from build123d import *

# Parameters (mm, degrees)
F1_DEPTH = 11.906
F3_DEPTH = 3.81
F5_DEPTH = 14.54711
F7_R     = 0.4


with BuildPart() as f1:
    # F0 (on Front) → F1 (new body)
    with BuildSketch(Plane.XZ):
        with BuildLine():
            Line((5.478281, 8.795274), (-5.478281, 8.795274))
            ThreePointArc((-5.478281, 8.795274), (-6.747731, 8.26945), (-7.273555, 7))
            Line((-7.273555, 7), (-7.273555, -7))
            ThreePointArc((-7.273555, -7), (-6.747731, -8.26945), (-5.478281, -8.795274))
            Line((-5.478281, -8.795274), (5.478281, -8.795274))
            ThreePointArc((5.478281, -8.795274), (6.747731, -8.26945), (7.273555, -7))
            Line((7.273555, -7), (7.273555, 7))
            ThreePointArc((7.273555, 7), (6.747731, 8.26945), (5.478281, 8.795274))
        make_face()
    extrude(amount=-F1_DEPTH)

    # F2 (on face) → F3 (join)
    with BuildSketch(Plane(origin=(0, 11.906, 0), x_dir=(-1, 0, 0), z_dir=(0, 1, 0))):
        with BuildLine():
            ThreePointArc((8.162555, 7), (7.376349, 8.898068), (5.478281, 9.684274))
            Line((5.478281, 9.684274), (-5.478281, 9.684274))
            ThreePointArc((-5.478281, 9.684274), (-7.376349, 8.898068), (-8.162555, 7))
            Line((-8.162555, 7), (-8.162555, -7))
            ThreePointArc((-8.162555, -7), (-7.376349, -8.898068), (-5.478281, -9.684274))
            Line((-5.478281, -9.684274), (5.478281, -9.684274))
            ThreePointArc((5.478281, -9.684274), (7.376349, -8.898068), (8.162555, -7))
            Line((8.162555, -7), (8.162555, 7))
        make_face()
    extrude(amount=F3_DEPTH)

    # F4 (on face) → F5 (cut, through all)
    with BuildSketch(Plane(origin=(-7.273555, 0, 0), x_dir=(0, -1, 0), z_dir=(-1, 0, 0))):
        Polygon((0, -3.496099), (0, 7), (0, 8.795274), (-3.105232, 8.795274), align=None)
    extrude(amount=-F5_DEPTH, mode=Mode.SUBTRACT)

    # F7
    f7_edges = [f1.edges().sort_by_distance(p)[0] for p in [
        (0, 3.105232, 8.795274),
        (6.757507, 2.969901, 8.259598),
        (7.273555, 1.325841, 1.75195),
        (7.273555, 0, -5.24805),
        (6.747731, 0, -8.26945),
        (0, 0, -8.795274),
        (-7.273555, 0, -5.24805),
        (-6.747731, 0, -8.26945),
        (-7.273555, 1.325841, 1.75195),
        (-6.757507, 2.969901, 8.259598),
    ]]
    fillet(f7_edges, radius=F7_R)


solid = f1.part
Model file for the job. Use its own axes, mm. A direction names the side the tool comes from. Give positions to 0.01 mm unless a question says otherwise; leave off trailing zeros. Order: outer loops, then holes, each group sorted by start corner. A loop starts at its lowest first (then second) coordinate and runs counter-clockwise, first axis right, second up. Notation, with made-up numbers: (17, 19.25) - (71, 19.25) arc R21 cw to (71, 53.25) - close; hole circle Ø3 at (18.5, 44). An arc over 180 degrees is marked (long way). Write item = value, one per line. Start each with the question number.
1. Cut at A-A, the plane y = 7. List the corners of the cut face in (x, z).
2. Drop flat-ended pins along their axis: P1, Ø9, axis at y = 7, z = 0.5, coming from the +X side; P2, Ø4, axis at x = -0.5, y = 8.5, coming from the +Z side; P3, Ø3, axis at x = -4.5, y = 1.5, coming from the -Z side. Give the stop position or say it passes through.
3. Which spindle directions (+Z, -Z, +X, -X, +Y, -Y) get a long thin tool onto all of the face, cutting with end or side? Do faces 1 (the flat face through (-7.274, 6, 0)), 2 (the cylindrical face through (6.762, 7.423, 8.255)), 3 (the cylindrical face through (-6.734, 7.423, 8.283)), 4 (the cylindrical face through (-6.762, 6.072, -8.255)), 5 (the flat face through (0, 8, 8.795)). Say none if no direction does.
4. Probe line 1 along X through (y, z) = (9.75, 1); line 2 along Z through (x, y) = (2.75, 3.5); line 3 along X through (y, z) = (13, 8.5). List the from-to ranges inside material, lowest first.
5. Cut at B-B, the plane x = 1.5. List the corners of the cut face in (y, z), and give its area (3 significant figures).
6. Cut at C-C, the plane z = -4.75. List the corners of the cut face in (x, y).
Taken from the geometry:
q1.outline = (-7.27, -7) arc R1.8 ccw to (-5.48, -8.8) - (5.48, -8.8) arc R1.8 ccw to (7.27, -7) - (7.27, 7) arc R1.8 ccw to (5.48, 8.8) - (-5.48, 8.8) arc R1.8 ccw to (-7.27, 7) - close
q2.P1 = 7.27
q2.P2 = 8.8
q2.P3 = -8.8
q3.face_1 = +Z, -Z, -X, -Y
q3.face_2 = +Z, +X, -Y
q3.face_3 = +Z, -X, -Y
q3.face_4 = -Z, -X, -Y
q3.face_5 = +Z, +X, -X, -Y
q4.line_1 = -7.27 to 7.27
q4.line_2 = -8.8 to 8.8
q4.line_3 = -7.7 to 7.7
q5.outline = (0, -8.4) arc R0.4 ccw to (0.4, -8.8) - (11.91, -8.8) - (11.91, -9.68) - (15.72, -9.68) - (15.72, 9.68) - (11.91, 9.68) - (11.91, 8.8) - (3.42, 8.8) arc R0.4 ccw to (3.03, 8.49) - (0, -3.5) - close
q5.area = 264 mm²
q6.outline = (-8.16, 11.91) - (-7.27, 11.91) - (-7.27, 0.4) arc R0.4 ccw to (-6.87, 0) - (6.87, 0) arc R0.4 ccw to (7.27, 0.4) - (7.27, 11.91) - (8.16, 11.91) - (8.16, 15.72) - (-8.16, 15.72) - close
